Geometry check sheet. Reference: the model listing, model coordinates, mm. A direction names the side the tool comes from. Give positions to 0.01 mm unless a question says otherwise; leave off trailing zeros. Loops run counter-clockwise (first coordinate to the right, second up) from the corner with the lowest first, then second, coordinate; pieces in that order, holes last. Notation, with made-up numbers: (-15.5, -8.5) -> (25.5, -8.5) arc R26 ccw to (25.5, 27.5) -> close; hole circle Ø6 at (53.5, 53.5). An arc over 180 degrees is marked (long way). Write item = value, one per line. Start each with the question number.
```python
from build123d import *

# Parameters (mm, degrees)
SKETCH1_R               = 11.5
BOSS_EXTRUDE1_DEPTH     = 18
SKETCH2_R               = 2.5
BOSS_EXTRUDE2_DEPTH     = 6
SKETCH3_R               = 11.5
BOSS_EXTRUDE3_DEPTH     = 4
FILLET1_R               = 2
CUT_EXTRUDE2_DEPTH      = 33.380549753
CUT_EXTRUDE2_DEPTH_BACK = 33.380549753
SKETCH5_R               = 6


with BuildPart() as part:
    # Sketch1 → Boss-Extrude1 (new body)
    with BuildSketch(Plane.XY):
        Circle(SKETCH1_R)
    extrude(amount=BOSS_EXTRUDE1_DEPTH)

    # Sketch2 → Boss-Extrude2 (add)
    with BuildSketch(Plane.XY.offset(18)):
        Circle(SKETCH2_R)
    extrude(amount=BOSS_EXTRUDE2_DEPTH)

    # Sketch3 → Boss-Extrude3 (add)
    with BuildSketch(Plane.XY.offset(24)):
        Circle(SKETCH3_R)
    extrude(amount=BOSS_EXTRUDE3_DEPTH)

    # Fillet1
    fillet1_edges = [part.edges().sort_by_distance(p)[0] for p in [
        (-11.5, 0, 24),
        (-11.5, 0, 28),
    ]]
    fillet(fillet1_edges, radius=FILLET1_R - 0.0001)  # a hair under: the kernel refuses the full size

    # Mirror1: part across plane


with BuildPart() as part_1:
    add(part.part)
    add(part.part.mirror(Plane.XY))

    # Sketch5 → Cut-Extrude2 (cut, two sides: drawn at the far end of the back side and taken through both)
    with BuildSketch(Plane(origin=(0, 0, 0), x_dir=(0, 0, -1), z_dir=(1, 0, 0)).offset(-CUT_EXTRUDE2_DEPTH_BACK)):
        Circle(SKETCH5_R)
    extrude(amount=CUT_EXTRUDE2_DEPTH + CUT_EXTRUDE2_DEPTH_BACK, mode=Mode.SUBTRACT)


solid = part_1.part
```
1) Tool access check on faces 1 (the flat face through (2, -2, 24)), 2 (the cylindrical face through (0, 0, 6)). Record the directions out of +Z, -Z, +X, -X, +Y, -Y that give a thin tool (end or side, any length) a straight path to the whole face; none if there is none.
2) Depth check by flat-ended pin: pin 1 Ø1 at (y, z) = (-6.5, 11.5) entering from -X; pin 2 Ø3 at (y, z) = (-5, -10) entering from -X; pin 3 Ø5 at (x, z) = (2, 9) entering from -Y; pin 4 Ø3 at (x, z) = (3.5, 8.5) entering from -Y. Enter the tip coordinate at first touch or a pass-through.
3) Section check C-C (z = 0). Enter the section's corners in (x, y).
4) Draft check along Z on faces 3 (the flat face through (0, 0, 28)), 4 (the flat face through (2, -2, -24)), 5 (the flat face through (0, 0, -28)). Enter one of: released by +Z, released by -Z, zero draft, split by the parting line, or undercut.
5) Section check D-D (x = -6.5). Give the number of separate pieces and of enclosed holes in the cut face, plus the area to 3 significant figures.
6) Thickness scan on line 1 (Z direction, x = 6.25, y = 0); line 2 (Z direction, x = 0.5, y = 0); line 3 (Z direction, x = -0.25, y = -4). Record the ranges inside material, lowest first.
Check result:
q1.face_1 = none
q1.face_2 = +X, -X
q2.pin_1 = -9.81
q2.pin_2 = -10.95
q2.pin_3 = -11.5
q2.pin_4 = -11.32
q3.outline = (-9.81, -6) arc R11.5 ccw to (9.81, -6) -> close; (-9.81, 6) -> (9.81, 6) arc R11.5 ccw to start
q4.face_3 = released by +Z
q4.face_4 = undercut
q4.face_5 = released by -Z
q5.separate_pieces = 3
q5.enclosed_holes = 1
q5.area = 713 mm2
q6.line_1 = -28 to -24, -18 to -6, 6 to 18, 24 to 28
q6.line_2 = -28 to -6, 6 to 28
q6.line_3 = -28 to -24, -18 to -4.47, 4.47 to 18, 24 to 28
